Read the model definition and answer for the solid it produces. Units are mm, in the model's axes. Coordinates: 2 decimals unless noted, no trailing zeros. Loops run counter-clockwise (first coordinate to the right, second up) from the corner with the lowest first, then second, coordinate; pieces in that order, holes last. Notation, with made-up numbers: (-16.75, 83) - (17.25, 83) arc R9 ccw to (17.25, 90) - close; hole circle Ø9 at (71.5, -6). An arc over 180 degrees is marked (long way). One line per question, with ' | ' between items. Start each with the question number.
```python
from build123d import *

# Parameters (mm, degrees)
BOSS_EXTRUDE1_DEPTH  = 7
F_2_5MM_CHAMFER_SIZE = 2.5
F_0_5MM_CHAMFER_SIZE = 0.5


with BuildPart() as part:
    # Sketch1 → Boss-Extrude1 (new body)
    with BuildSketch(Plane.XY):
        with BuildLine():
            Line((-32.037980617, 40.14916039), (-14.889638473, 37.125444996))
            ThreePointArc((-14.889638473, 37.125444996), (0, 40), (14.889638473, 37.125444996))
            Line((14.889638473, 37.125444996), (32.037980617, 40.14916039))
            Line((32.037980617, 40.14916039), (34.5, 43.083280834))
            Line((34.5, 43.083280834), (34.5, 150))
            Line((34.5, 150), (-34.5, 150))
            Line((-34.5, 150), (-34.5, 43.083280834))
            Line((-34.5, 43.083280834), (-32.037980617, 40.14916039))
        make_face()
    extrude(amount=BOSS_EXTRUDE1_DEPTH)

    # 2,5mm Chamfer
    f_2_5mm_chamfer_edges = [part.edges().sort_by_distance(p)[0] for p in [
        (23.463809545, 38.637302693, 7),
        (33.268990309, 41.616220612, 7),
        (34.5, 96.541640417, 7),
        (-34.5, 96.541640417, 7),
        (-33.268990309, 41.616220612, 7),
        (-23.463809545, 38.637302693, 7),
        (0, 40, 7),
    ]]
    chamfer(f_2_5mm_chamfer_edges, length=F_2_5MM_CHAMFER_SIZE)

    # 0,5mm Chamfer
    f_0_5mm_chamfer_edges = [part.edges().sort_by_distance(p)[0] for p in [
        (-34.5, 150, 2.25),
        (0, 150, 7),
        (34.5, 150, 2.25),
        (33.25, 150, 5.75),
        (-33.25, 150, 5.75),
    ]]
    chamfer(f_0_5mm_chamfer_edges, length=F_0_5MM_CHAMFER_SIZE)


solid = part.part
```
1) The part is cut by section C-C on x = 25. Write down the section's boundary in (y, z).
2) The part is cut by section B-B on x = -27.5. Write down the section's boundary in (y, z), and give its area (3 significant figures).
3) Given pin 1 Ø1 at (x, z) = (-27, 3) entering from -Y, flat-ended and moving along its own axis, determine where the tip first touches the part or whether it passes through.
4) The part is cut by section A-A on z = 2. Write down the section's boundary in (x, y), and give its area (3 significant figures).
5) Find the intervals of material crossed by line 1 along Y through (x, z) = (-2.5, 4.75); line 2 along Y through (x, z) = (21.5, 0.75); line 3 along X through (y, z) = (113.5, 5.5), in increasing order. Write a range as from..to.
6) The mould has two halves that part along X. Classify faces 1 (the flat face through (0, 150, 3)), 2 (the conical face through (-0.2, 40.7, 5.2)), 3 (the flat face through (33.252, 41.596, 2.218)), 4 (the cylindrical face through (0, 40, 2)): released by +X, released by -X, zero draft, split by the parting line, or undercut.
Answer below:
1) outline: (38.91, 0) - (150, 0) - (150, 6.5) - (149.5, 7) - (41.45, 7) - (38.91, 4.5) - close
2) outline: (39.35, 0) - (150, 0) - (150, 6.5) - (149.5, 7) - (41.89, 7) - (39.35, 4.5) - close | area: 771 mm2
3) pin 1: y = 39.17
4) outline: (-34.5, 43.08) - (-32.04, 40.15) - (-14.89, 37.13) arc R40 cw to (14.89, 37.13) - (32.04, 40.15) - (34.5, 43.08) - (34.5, 149.5) - (34, 150) - (-34, 150) - (-34.5, 149.5) - close | area: 7,660 mm2
5) line 1: 40.17..150 | line 2: 38.29..150 | line 3: -33.5..33.5
6) face 1: zero draft | face 2: undercut | face 3: released by +X | face 4: undercut
